from build123d import *

# Parameters (mm, degrees)
F0_R     = 15
F0_W     = 2.201593481
F0_H     = 1
F0_W_2   = 0.7
F0_H_2   = 2
F0_W_3   = 0.611269173
F0_H_3   = 0.7
F0_W_4   = 0.547691976
F0_W_5   = 0.5653050612
F1_DEPTH = 1


# Not quite as in the source:
# - a fillet or chamfer that OpenCascade refuses, or shapes differently, is made with other operations: its cross-section is extruded or revolved along the edge and cut away or added
# - a feature names something its author has since deleted; it is built from what else it names


with BuildPart() as f1:
    # F0 (on Top) → F1 (new body)
    with BuildSketch(Plane.XY):
        Circle(F0_R)
        with Locations((-8.9021953754, -9.5)):
            Rectangle(F0_W, F0_H, mode=Mode.SUBTRACT)
        with Locations((-10.9492010795, -7)):
            Rectangle(F0_W_2, F0_H_2, mode=Mode.SUBTRACT)
        with Locations((-10.9935664929, -4)):
            Rectangle(F0_W_3, F0_H_2, mode=Mode.SUBTRACT)
        with Locations((-8.9021953754, -5.35)):
            Rectangle(F0_W, F0_H_3, mode=Mode.SUBTRACT)
        with Locations((-8.9021953754, -2.65)):
            Rectangle(F0_W, F0_H_3, mode=Mode.SUBTRACT)
        with Locations((-6.7348206503, -7)):
            Rectangle(F0_W_4, F0_H_2, mode=Mode.SUBTRACT)
        with Locations((-6.7848820763, -4)):
            Rectangle(F0_W_5, F0_H_2, mode=Mode.SUBTRACT)
        with Locations((8.9021953754, -9.5)):
            Rectangle(F0_W, F0_H, mode=Mode.SUBTRACT)
        with Locations((6.7348206503, -7)):
            Rectangle(F0_W_4, F0_H_2, mode=Mode.SUBTRACT)
        with Locations((6.7848820763, -4)):
            Rectangle(F0_W_5, F0_H_2, mode=Mode.SUBTRACT)
        with Locations((10.9492010795, -7)):
            Rectangle(F0_W_2, F0_H_2, mode=Mode.SUBTRACT)
        with Locations((8.9021953754, -5.35)):
            Rectangle(F0_W, F0_H_3, mode=Mode.SUBTRACT)
        with Locations((10.9935664929, -4)):
            Rectangle(F0_W_3, F0_H_2, mode=Mode.SUBTRACT)
        with Locations((8.9021953754, -2.65)):
            Rectangle(F0_W, F0_H_3, mode=Mode.SUBTRACT)
        with Locations((-8.9021953754, 2.65)):
            Rectangle(F0_W, F0_H_3, mode=Mode.SUBTRACT)
        with Locations((-10.9935664929, 4)):
            Rectangle(F0_W_3, F0_H_2, mode=Mode.SUBTRACT)
        with Locations((-8.9021953754, 5.35)):
            Rectangle(F0_W, F0_H_3, mode=Mode.SUBTRACT)
        with Locations((-10.9492010795, 7)):
            Rectangle(F0_W_2, F0_H_2, mode=Mode.SUBTRACT)
        with Locations((-2.9021953754, 2.65)):
            Rectangle(F0_W, F0_H_3, mode=Mode.SUBTRACT)
        with Locations((-6.7848820763, 4)):
            Rectangle(F0_W_5, F0_H_2, mode=Mode.SUBTRACT)
        with Locations((-4.9935664929, 4)):
            Rectangle(F0_W_3, F0_H_2, mode=Mode.SUBTRACT)
        with Locations((-6.7348206503, 7)):
            Rectangle(F0_W_4, F0_H_2, mode=Mode.SUBTRACT)
        with Locations((-4.9492010795, 7)):
            Rectangle(F0_W_2, F0_H_2, mode=Mode.SUBTRACT)
        with Locations((-2.9021953754, 5.35)):
            Rectangle(F0_W, F0_H_3, mode=Mode.SUBTRACT)
        with Locations((-0.7848820763, 4)):
            Rectangle(F0_W_5, F0_H_2, mode=Mode.SUBTRACT)
        with Locations((-0.7348206503, 7)):
            Rectangle(F0_W_4, F0_H_2, mode=Mode.SUBTRACT)
        Polygon((-10.0029921159, 9), (-7.8013986349, 9), (-7.8024366548, 8.2387067378), (-10.0029921159, 8.2387067378), align=None, mode=Mode.SUBTRACT)
        Polygon((-1.8024366548, 8.2387067378), (-4.0029921159, 8.2387067378), (-4.0029921159, 9), (-1.8013986349, 9), align=None, mode=Mode.SUBTRACT)
        with Locations((3.0978046246, 2.65)):
            Rectangle(F0_W, F0_H_3, mode=Mode.SUBTRACT)
        with Locations((1.0064335071, 4)):
            Rectangle(F0_W_3, F0_H_2, mode=Mode.SUBTRACT)
        with Locations((3.0978046246, 5.35)):
            Rectangle(F0_W, F0_H_3, mode=Mode.SUBTRACT)
        with Locations((1.0507989205, 7)):
            Rectangle(F0_W_2, F0_H_2, mode=Mode.SUBTRACT)
        with Locations((5.2151179237, 4)):
            Rectangle(F0_W_5, F0_H_2, mode=Mode.SUBTRACT)
        with Locations((6.7848820763, 4)):
            Rectangle(F0_W_5, F0_H_2, mode=Mode.SUBTRACT)
        with Locations((5.2651793497, 7)):
            Rectangle(F0_W_4, F0_H_2, mode=Mode.SUBTRACT)
        with Locations((6.7348206503, 7)):
            Rectangle(F0_W_4, F0_H_2, mode=Mode.SUBTRACT)
        with Locations((8.9021953754, 2.65)):
            Rectangle(F0_W, F0_H_3, mode=Mode.SUBTRACT)
        with Locations((8.9021953754, 5.35)):
            Rectangle(F0_W, F0_H_3, mode=Mode.SUBTRACT)
        with Locations((10.9935664929, 4)):
            Rectangle(F0_W_3, F0_H_2, mode=Mode.SUBTRACT)
        with Locations((10.9492010795, 7)):
            Rectangle(F0_W_2, F0_H_2, mode=Mode.SUBTRACT)
        Polygon((4.1975633452, 8.2387067378), (1.9970078841, 8.2387067378), (1.9970078841, 9), (4.1986013651, 9), align=None, mode=Mode.SUBTRACT)
        Polygon((10.0029921159, 9), (10.0029921159, 8.2387067378), (7.8024366548, 8.2387067378), (7.8013986349, 9), align=None, mode=Mode.SUBTRACT)
    extrude(amount=F1_DEPTH)

    # F2: fillet of radius 1 on 1 edges, made by hand

    # F2_s1 → F2_t2 (revolve, cut)
    with BuildSketch(Plane.XZ):
        with BuildLine():
            ThreePointArc((15, 0), (14.7071067812, 0.7071067812), (14, 1))
            Line((14, 1), (15, 1))
            Line((15, 1), (15, 0))
        make_face()
    revolve(axis=Axis((0, 0, 1), (0, 0, 1)), mode=Mode.SUBTRACT)


solid = f1.part
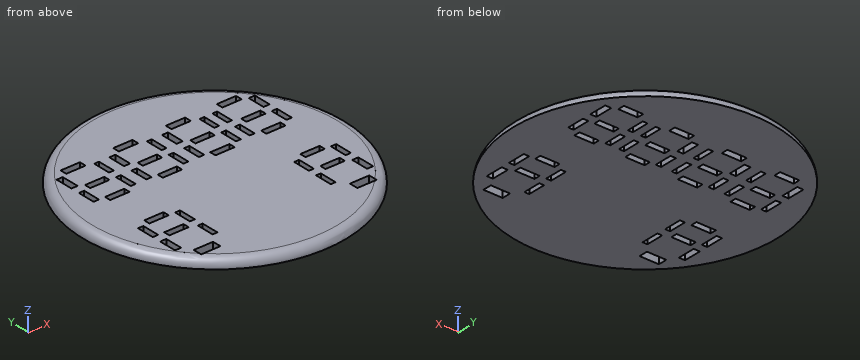
Design review of the part built by this model. Coordinates are the model's own, in mm. Coordinates: 2 decimals unless noted, no trailing zeros.
Item 1: Wall thickness on L1, parallel to X at y = -2.5, z = 0.2; L2, parallel to Y at x = -3.5, z = 0.1; L3, parallel to Y at x = 2.5, z = 0.25: over which ranges is each line inside the solid? List them lowest first.
Completed:
L1: x = -14.77 to -10, -7.8 to 7.8, 10 to 14.77
L2: y = -14.58 to 2.3, 3 to 5, 5.7 to 8.24, 9 to 14.58
L3: y = -14.76 to 2.3, 3 to 5, 5.7 to 8.24, 9 to 14.76
Item 2: Add section A-A (z = 0.6). Give the number of separate pieces and of enclosed holes in the cut face, and give its area (3 significant figures).
Completed:
separate pieces: 1
enclosed holes: 42
area: 629 mm2
Item 3: Clearance check with flat-ended pins moving along their axes: pin 1 (0.5 mm diameter, centred on y = 3.5, z = 0.5, fed in from -X); pin 2 (0.5 mm diameter, centred on y = 7.5, z = 0.5, fed in from -X); pin 3 (0.5 mm diameter, centred on y = -9.5, z = 0.5, fed in from -X). State where each tip first meets the part, or that it passes through.
Completed:
pin 1: stops at x = -14.57
pin 2: stops at x = -13.03
pin 3: stops at x = -11.69
